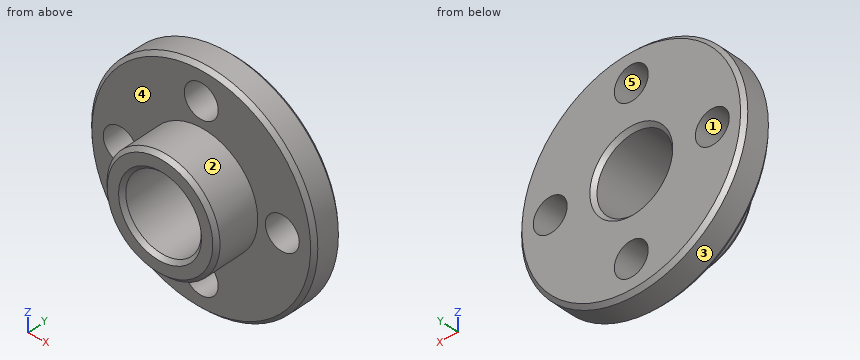
Autodesk Inventor part; units mm, degrees
ref_plane "YZ Plane" through (0, 0, 0) normal (1, 0, 0) x (0, 1, 0)
ref_plane "XZ Plane" through (0, 0, 0) normal (0, 1, 0) x (-1, 0, 0)
ref_plane "XY Plane" through (0, 0, 0) normal (0, 0, 1) x (1, 0, 0)
sketch "Esboço1" plane through (0, 0, 0) normal (0, 0, 1) x (1, 0, 0)
  line L0 (-18, 0) -> (3, 0) construction
  line L1 (0, -8) -> (0, 6) construction
  line L2 (-5, 4) -> (-5, -6)
  line L3 (-5, -6) -> (-7.5, -6)
  line L4 (-7.5, -6) -> (-7.5, 0)
  line L5 (-7.5, 0) -> (-15, 0)
  line L6 (-15, 0) -> (-15, 4)
  line L7 (-15, 4) -> (-5, 4)
  point P0 (0, 0)
  dimension "d0" = 30
  dimension "d1" = 10
  dimension "d2" = 4
  dimension "d3" = 10
  dimension "d4" = 15
revolve "Revolução1" add sketch "Esboço1" angle 360 about axis through (0, -10, 0) along (0, 1, 0)
sketch "Esboço2" plane through (0, 4, 0) normal (0, 1, 0) x (1, 0, 0)
  line L0 (-21, 0) -> (21, 0) construction
  line L1 (0, 21) -> (0, -21) construction
  circle A0 centre (0, 0) radius 10.75 construction
  circle A1 centre (0, -10.75) radius 3.5
  circle A2 centre (0, -10.75) radius 2.25
  point P0 (-10.75, 0)
  point P1 (10.75, 0)
  point P2 (0, 10.75)
  dimension "d6" = 21.5
  dimension "d7" = 7
  dimension "d8" = 4.5
hole "Furo1" at (-10.75, 4, 0) at (10.75, 4, 0) at (0, 4, 10.75) at (0, 4, -10.75) direction (0, -1, 0) diameter 4.5 end through all
chamfer "Chanfro1" distance 0.5 angle 45 5 edges at (15, 4, 0) (15, 0, 0) (5, 4, 0) (5, -6, 0) (7.5, -6, 0)
properties part number "Compensador Limitador" material "Aço SAE 1045"
Geometry check sheet. Reference: the model listing, model coordinates, mm. Face numbers are marked on the shaded views. A direction names the side the tool comes from. Round coordinates to 2 decimals unless told otherwise and drop trailing zeros. Loops run counter-clockwise (first coordinate to the right, second up) from the corner with the lowest first, then second, coordinate; pieces in that order, holes last. Notation, with made-up numbers: (48.5, -38) - (72.5, -38) arc R32 cw to (72.5, -4) - close; hole circle Ø4 at (40, 25). An arc over 180 degrees is marked (long way). Use a Markdown table: item, result.
Q1. Material ranges on line 1 (Z direction, x = 0, y = 1.1); line 2 (Z direction, x = 0, y = -3); line 3 (Y direction, x = -3.5, z = -9), recorded low to high.
Solutions:
| item | result |
|---|---|
| line 1 | z = -15 to -13, -8.5 to -5, 5 to 8.5, 13 to 15 |
| line 2 | z = -7.5 to -5, 5 to 7.5 |
| line 3 | y = 0 to 4 |
Q2. Cross-section at A-A on x = 0. State how many separate pieces and enclosed holes the cut face has, plus the area to 4 significant figures.
Solutions:
| item | result |
|---|---|
| separate pieces | 4 |
| enclosed holes | 0 |
| area | 72.75 mm2 |
Q3. Cross-section at C-C on y = -1. Record the cut outline in (x, z).
Solutions:
| item | result |
|---|---|
| outline | circle Ø15 at (0, 0); hole circle Ø10 at (0, 0) |
Q4. Draft check along X on the marked faces 3, 4 and 5. Enter one of: released by +X, released by -X, zero draft, split by the parting line, or undercut.
Solutions:
| item | result |
|---|---|
| face 3 | split by the parting line |
| face 4 | zero draft |
| face 5 | undercut |
Q5. Go/stop test with flat-tipped pins: P1, Ø2, axis at y = 0, z = -6, coming from the -X side; P2, Ø4, axis at x = -10.75, z = 0, coming from the -Y side; P3, Ø5, axis at x = 0, z = -10.75, coming from the -Y side; P4, Ø5, axis at y = -4, z = 9, coming from the +X side. Record where each tip stops, or that it passes through.
Solutions:
| item | result |
|---|---|
| P1 | stops at x = -14.09 |
| P2 | passes through |
| P3 | stops at y = 0 |
| P4 | stops at x = 3.74 |
Q6. Access from +Z, -Z, +X, -X, +Y, -Y to the whole of each face (thin tool, end or side, straight path). Record for the marked faces 1 and 2.
Solutions:
| item | result |
|---|---|
| face 1 | +Y, -Y |
| face 2 | -Y |
